Answer from the drawing. Dimensions are ordinates in mm from the lowest x, y and z of the part. Give positions to 0.01 mm unless a question says otherwise; leave off trailing zeros. Loops run counter-clockwise (first coordinate to the right, second up) from the corner with the lowest first, then second, coordinate; pieces in that order, holes last.
(1) Find section C-C, the plane z = 114.3. Write down the section's boundary in (x, y) (3 decimals).
(2) Find section A-A, the plane z = 25.4. Write down the section's boundary in (x, y) (3 decimals).
(3) Find section B-B, the plane y = 3.75. Write down the section's boundary in (x, z) (3 decimals).
(4) Straight lines are drawn through the part: probe 1 along X at (y, z) = (3, 114.3) (3 decimals); probe 2 along Z at (x, y) = (60, 5.5); probe 3 along X at (y, z) = (1, 35). For each, find the intervals that lie inside material, in ascending order.
(5) Find section D-D, the plane z = 10. Write down the section's boundary in (x, y).
(6) This flat-tipped pin is pushed along its axis until it touches: P1, Ø5, axis at x = 31.75, z = 66.675, coming from the -Y side. Where does it stop, or does it pass through?
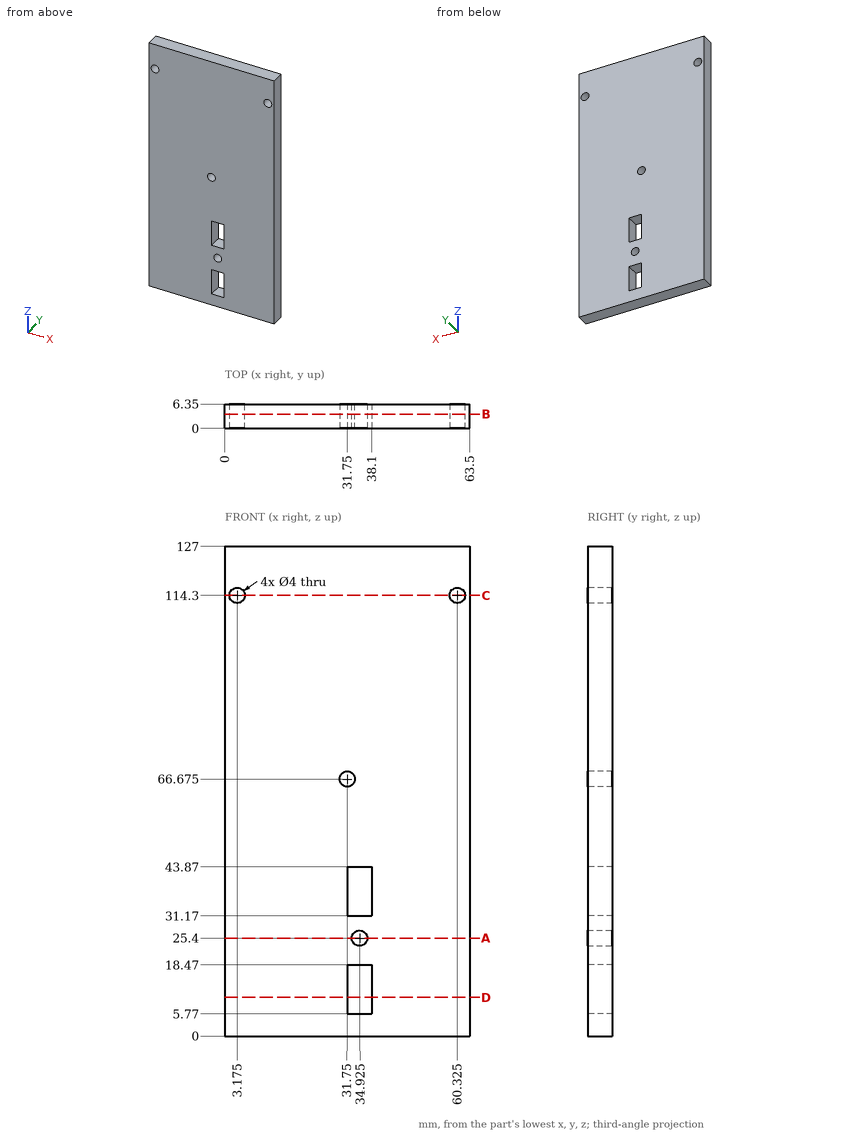
Entries:
1. outline: (0, 0) - (1.175, 0) - (1.175, 6.35) - (0, 6.35) - close; (5.175, 0) - (58.325, 0) - (58.325, 6.35) - (5.175, 6.35) - close; (62.325, 0) - (63.5, 0) - (63.5, 6.35) - (62.325, 6.35) - close
2. outline: (0, 0) - (32.925, 0) - (32.925, 6.35) - (0, 6.35) - close; (36.925, 0) - (63.5, 0) - (63.5, 6.35) - (36.925, 6.35) - close
3. outline: (0, 0) - (63.5, 0) - (63.5, 127) - (0, 127) - close; hole circle Ø4 at (3.175, 114.3); hole circle Ø4 at (31.75, 66.675); hole (31.75, 5.77) - (38.1, 5.77) - (38.1, 18.47) - (31.75, 18.47) - close; hole (31.75, 31.17) - (38.1, 31.17) - (38.1, 43.87) - (31.75, 43.87) - close; hole circle Ø4 at (34.925, 25.4); hole circle Ø4 at (60.325, 114.3)
4. probe 1: x = 0 to 1.175, 5.175 to 58.325, 62.325 to 63.5
4. probe 2: z = 0 to 112.33, 116.27 to 127
4. probe 3: x = 0 to 31.75, 38.1 to 63.5
5. outline: (0, 0) - (31.75, 0) - (31.75, 6.35) - (0, 6.35) - close; (38.1, 0) - (63.5, 0) - (63.5, 6.35) - (38.1, 6.35) - close
6. P1: stops at y = 0
